The figure shows three views and two pictorial views of one solid part (mm, origin at its lowest corner). Answer the questions. A direction names the side the tool comes from. Give positions to 0.01 mm unless a question says otherwise; leave off trailing zeros. Order: outer loops, then holes, each group sorted by start corner. A loop starts at its lowest first (then second) coordinate and runs counter-clockwise, first axis right, second up. Notation, with made-up numbers: (-34, -10) - (-21, -10) arc R25 ccw to (-21, 5) - close; hole circle Ø3 at (51.25, 65). An arc over 180 degrees is marked (long way). Answer as a JSON object with one key per item and string values. Group by question number.
Q1. Consider line 1 (X direction, y = 22, z = 12.5); line 2 (X direction, y = 34, z = 29). Determine where each line is inside the solid, lowest interval first.
Q2. For the marked faces 5 and 6, determine the directions among +Z, -Z, +X, -X, +Y, -Y from which every point of the face is accessible in a straight line to the end or side of a thin tool.
Q3. A cutting plane is placed at D-D, the plane z = 25. Give the vertices of the cut face in (x, y).
Q4. A cutting plane is placed at C-C, the plane z = 7. Give the vertices of the cut face in (x, y).
Q5. Given pin 1 (7.5 mm diameter, centred on x = 35.91, y = 25.59, fed in from -Z); pin 2 (1 mm diameter, centred on x = 50, y = 19, fed in from +Z); pin 3 (4 mm diameter, centred on x = 25.59, y = 35.91, fed in from +Z); pin 4 (3 mm diameter, centred on y = 26, z = 25.5, fed in from -X), each flat-ended and moving along its own axis, determine where each tip first touches the part or whether it passes through.
Q6. The mould has two halves that part along Y. Classify the marked faces 1, 2, 3 and 4: released by +Y, released by -Y, zero draft, split by the parting line, or undercut.
Q7. A cutting plane is placed at B-B, the plane y = 45. Give the vertices of the cut face in (x, z).
Q8. A cutting plane is placed at A-A, the plane x = 40. Give the vertices of the cut face in (y, z), and give its area (3 significant figures).
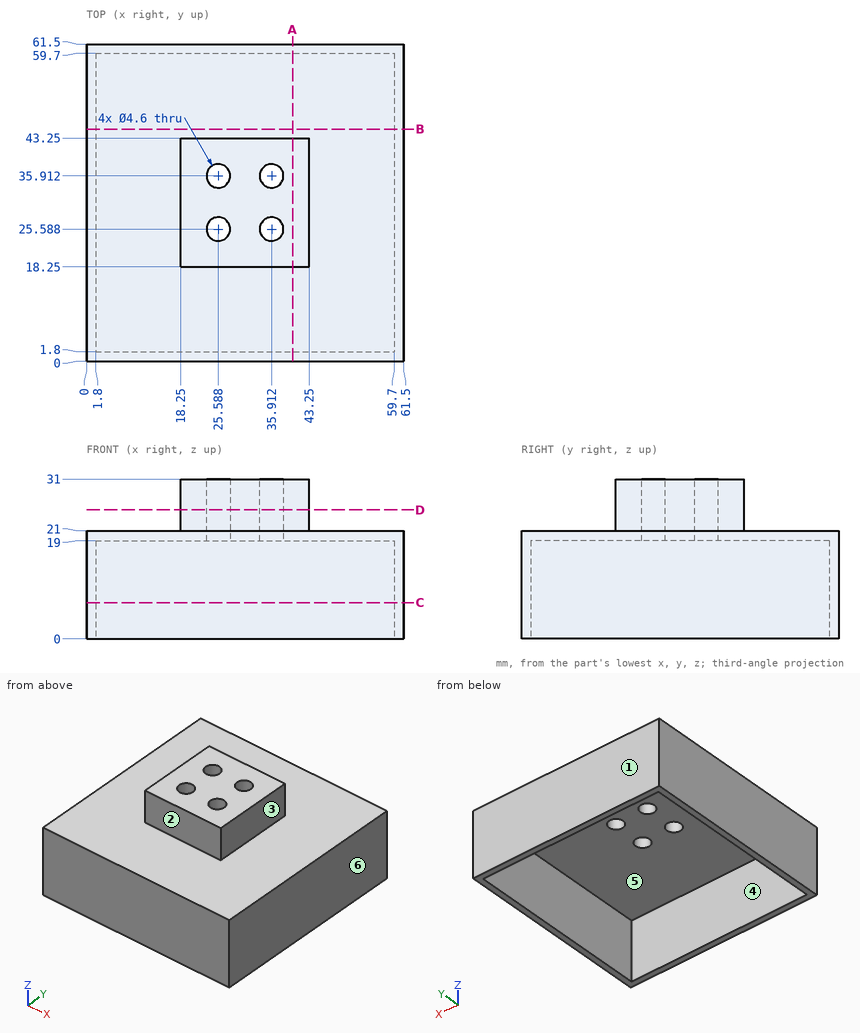
Reply:
{
 "1": {"line 1": "x = 0 to 1.8, 59.7 to 61.5", "line 2": "x = 18.25 to 24.31, 26.87 to 34.63, 37.19 to 43.25"},
 "2": {"face 5": "-Z", "face 6": "+Z, -Z, +X, +Y, -Y"},
 "3": {"outline": "(18.25, 18.25) - (43.25, 18.25) - (43.25, 43.25) - (18.25, 43.25) - close; hole circle Ø4.6 at (25.59, 25.59); hole circle Ø4.6 at (25.59, 35.91); hole circle Ø4.6 at (35.91, 25.59); hole circle Ø4.6 at (35.91, 35.91)"},
 "4": {"outline": "(0, 0) - (61.5, 0) - (61.5, 61.5) - (0, 61.5) - close; hole (1.8, 1.8) - (59.7, 1.8) - (59.7, 59.7) - (1.8, 59.7) - close"},
 "5": {"pin 1": "stops at z = 19", "pin 2": "stops at z = 21", "pin 3": "passes through", "pin 4": "stops at x = 18.25"},
 "6": {"face 1": "released by +Y", "face 2": "released by -Y", "face 3": "zero draft", "face 4": "undercut"},
 "7": {"outline": "(0, 0) - (1.8, 0) - (1.8, 19) - (59.7, 19) - (59.7, 0) - (61.5, 0) - (61.5, 21) - (0, 21) - close"},
 "8": {"outline": "(0, 0) - (1.8, 0) - (1.8, 19) - (59.7, 19) - (59.7, 0) - (61.5, 0) - (61.5, 21) - (43.25, 21) - (43.25, 31) - (18.25, 31) - (18.25, 21) - (0, 21) - close", "area": "441 mm^2"}
}
